Here's how the part is built. I have some questions about the finished solid (model axes, mm). Coordinates: 2 decimals unless noted, no trailing zeros. Loops run counter-clockwise (first coordinate to the right, second up) from the corner with the lowest first, then second, coordinate; pieces in that order, holes last. Notation, with made-up numbers: (-11.75, -18.5) -> (-2.75, -18.5) arc R25 ccw to (-2.75, -4.5) -> close; hole circle Ø1 at (-1.5, -9). An arc over 180 degrees is marked (long way). Answer as a JSON object with one key per item and string values. Group by question number.
1) I want a section at C-C (y = 11.5). Write out the boundary of the cut face in (x, z).
2) I'm going to push flat-ended pins straight in: pin 1 (12 mm diameter, centred on x = 19, y = 22, fed in from -Z); pin 2 (2 mm diameter, centred on y = 19.5, z = -0.5, fed in from +X); pin 3 (12 mm diameter, centred on y = -18.5, z = 5.5, fed in from +X). Where does each tip first touch, or does it pass through?
3) I want a section at A-A (x = 0). Write out the boundary of the cut face in (y, z).
4) I want a section at D-D (x = 16.5). Write out the boundary of the cut face in (y, z).
5) I want a section at B-B (z = 0). Write out the boundary of the cut face in (x, y), then the cut area to 3 significant figures.
6) I need wall thicknesses on probe 1 along X at (y, z) = (0.4, 0); probe 2 along Z at (x, y) = (-13.5, 0). Which ranges of each line are inside material? Lowest first, please. Write a range as [from, to].
```python
from build123d import *

# Parameters (mm, degrees)
SKETCH1_R           = 38.1
BOSS_EXTRUDE1_DEPTH = 50.827459459
SHELL2_T            = 3.175
REVOLVE1_ANGLE      = 180
SCALE1_SCALE        = 0.615384615


# Read off the part's stored shape, not the designer's step: Shell4
with BuildPart() as part:
    # Sketch1 → Boss-Extrude1 (new body)
    with BuildSketch(Plane(origin=(0, 0, 0), x_dir=(1, 0, 0), z_dir=(0, 1, 0))):
        with Locations(Location((0, 0, 0), (0, 0, 90))):
            Circle(SKETCH1_R)
    extrude(amount=BOSS_EXTRUDE1_DEPTH)

    # Shell2
    shell2_openings = [part.faces().sort_by_distance(p)[0] for p in [
        (0, 50.827459459, 0),
    ]]
    offset(amount=SHELL2_T, openings=shell2_openings, kind=Kind.INTERSECTION)

    # Sketch5 → Revolve1 (revolve)
    with BuildSketch(Plane.XZ.offset(3.175)):
        with BuildLine():
            Line((-40.445113765, 8.235192624), (40.445113765, -8.235192624))
            ThreePointArc((40.445113765, -8.235192624), (-8.235192624, -40.445113765), (-40.445113765, 8.235192624))
        make_face()
    revolve(axis=Axis((-40.445113765, -3.175, 8.235192624), (-0.979893731431563, 0, 0.19952011202164077)), revolution_arc=REVOLVE1_ANGLE)

    # Shell4 outline → Shell4 (revolve, cut)
    with BuildSketch(Plane.XY):
        with BuildLine():
            ThreePointArc((0, -41.275), (26.940768377, -30.11576835), (38.1, -3.174999962))
            Line((38.1, -3.174999962), (38.1, 0))
            Line((38.1, 0), (0, 0))
            Line((0, 0), (0, -41.275))
        make_face()
    revolve(axis=Axis((0, 0, 0), (0, 1, 0)), mode=Mode.SUBTRACT)


with BuildPart() as part_1:
    # Scale1: scaled about (-2e-09, 3.96741665, 0)
    add(part.part.scale(SCALE1_SCALE).moved(Location((-1e-09, 1.525929481, 0))))


solid = part_1.part
```
Determined:
{
 "1": {"outline": "circle Ø50.8 at (0, 0); hole circle Ø46.89 at (0, 0)"},
 "2": {"pin 1": "z = -21.82", "pin 2": "x = 25.4", "pin 3": "x = 21.89"},
 "3": {"outline": "(-0.43, -25.4) -> (32.8, -25.4) -> (32.8, -23.45) -> (-0.43, -23.45) arc R23.45 cw to (-0.43, 23.45) -> (32.8, 23.45) -> (32.8, 25.4) -> (-0.43, 25.4) arc R25.4 ccw to start"},
 "4": {"outline": "(-0.43, -19.31) -> (32.8, -19.31) -> (32.8, -16.66) -> (-0.43, -16.66) arc R16.66 cw to (-0.43, 16.66) -> (32.8, 16.66) -> (32.8, 19.31) -> (-0.43, 19.31) arc R19.31 ccw to start"},
 "5": {"outline": "(-25.4, -0.43) arc R25.4 ccw to (25.4, -0.43) -> (25.4, 32.8) -> (23.45, 32.8) -> (23.45, -0.43) arc R23.45 cw to (-23.45, -0.43) -> (-23.45, 32.8) -> (-25.4, 32.8) -> close", "area": "280 mm^2"},
 "6": {"probe 1": "[-25.4, -23.45], [23.45, 25.4]", "probe 2": "[-21.52, -19.17], [19.17, 21.52]"}
}
